from build123d import *

# Parameters (mm, degrees)
F1_DEPTH = 10
F3_DEPTH = 45
F4_W     = 2.981
F4_H     = 5
F4_W_2   = 1.6583123952
F5_DEPTH = 25
F6_R     = 2.49999
F8_DEPTH = 10
F9_R     = 2.5


# Not quite as in the source:
# - a fillet or chamfer is up to 0.001 mm smaller than in the source, because OpenCascade refuses the exact size
# - ends of sketch curves that miss each other by under 0.0002 mm in the source are joined


with BuildPart() as f1:
    # F0 (on Top) → F1 (new body)
    with BuildSketch(Plane.XY):
        with BuildLine():
            Line((70, 0), (10, 0))
            ThreePointArc((10, 0), (2.9289321881, -2.9289321881), (0, -10))
            Line((0, -10), (0, -40))
            ThreePointArc((0, -40), (2.9289321881, -47.0710678119), (10, -50))
            Line((10, -50), (70, -50))
            ThreePointArc((70, -50), (77.0710678119, -47.0710678119), (80, -40))
            Line((80, -40), (80, -10))
            ThreePointArc((80, -10), (77.0710678119, -2.9289321881), (70, 0))
        make_face()
    extrude(amount=F1_DEPTH)

    # F2 (on face) → F3 (cut)
    with BuildSketch(Plane.XZ.offset(50)):
        with BuildLine():
            ThreePointArc((40.8291561976, 0), (41.3216910184, 0.5406814173), (41.5, 1.25))
            ThreePointArc((41.5, 1.25), (39.2906814173, 2.5716910184), (39.1708438024, 0))
            Line((39.1708438024, 0), (40.8291561976, 0))
        make_face()
    extrude(amount=-F3_DEPTH, mode=Mode.SUBTRACT)

    # F4 (on face) → F5 (cut)
    with BuildSketch(Plane(origin=(0, 0, 0), x_dir=(1, 0, 0), z_dir=(0, 0, -1))):
        with Locations((37.6803438024, 7.5)):
            Rectangle(F4_W, F4_H)
        with Locations((40, 7.5)):
            Rectangle(F4_W_2, F4_H)
        with Locations((42.3196561976, 7.5)):
            Rectangle(F4_W, F4_H)
    extrude(amount=-F5_DEPTH, mode=Mode.SUBTRACT)

    # F6 (radius 2.5 in the source; OpenCascade refuses exactly that, so slightly less here)
    f6_edges = [f1.edges().sort_by_distance(p)[0] for p in [
        (36.189844, -5, 5),
        (43.810156, -5, 5),
        (43.810156, -10, 5),
        (36.189844, -10, 5),
    ]]
    fillet(f6_edges, radius=F6_R)

    # F7 (on face) → F8 (join)
    with BuildSketch(Plane.XY.offset(10)):
        Polygon((35.1898438024, -11), (40, -11), (44.8101561976, -11), (44.8101561976, -4), (35.1898438024, -4), align=None)
        with BuildLine():
            ThreePointArc((38.6898338024, -10), (36.9220739205, -9.2677698819), (36.1898438024, -7.50001))
            ThreePointArc((36.1898438024, -7.50001), (36.9220739205, -5.7322301181), (38.6898338024, -5))
            Line((38.6898338024, -5), (41.3101661976, -5))
            ThreePointArc((41.3101661976, -5), (43.0779260795, -5.7322301181), (43.8101561976, -7.49999))
            ThreePointArc((43.8101561976, -7.49999), (43.0779260795, -9.2677698819), (41.3101661976, -10))
            Line((41.3101661976, -10), (38.6898338024, -10))
        make_face(mode=Mode.SUBTRACT)
    extrude(amount=F8_DEPTH)

    # F9
    f9_edges = [f1.edges().sort_by_distance(p)[0] for p in [
        (44.810156, -4, 15),
        (35.189844, -4, 15),
        (35.189844, -11, 15),
        (44.810156, -11, 15),
    ]]
    fillet(f9_edges, radius=F9_R)


solid = f1.part
Geometry: final body of the model. Coordinates: model frame, mm. A direction names the side the tool comes from. Round coordinates to 2 decimals unless told otherwise and drop trailing zeros. Loops run counter-clockwise (first coordinate to the right, second up) from the corner with the lowest first, then second, coordinate; pieces in that order, holes last.
Q1. Pin query (flat end, axial travel): P1, Ø8, axis at y = -17.5, z = 12.5, coming from the +X side; P2, Ø3, axis at x = 39.5, z = 12.5, coming from the +Y side; P3, Ø12, axis at x = 28.5, y = -36, coming from the +Z side; P4, Ø1.6, axis at y = -7.5, z = 14, coming from the +X side. Return the tip coordinate at first contact, or that it passes through.
Q2. Section C-C on x = 9. Return loops of the section in (y, z), plus the area to 3 significant figures.
Q3. Access query for faces 4 (the cylindrical face through (35.903, -4.752, 15.07)), 5 (the cylindrical face through (35.942, -10.287, 15.07)), 6 (the flat face through (35.19, -7, 15)), 7 (the flat face through (44.81, -8, 15)), 8 (the flat face through (40, -10, 11)). Directions: +Z, -Z, +X, -X, +Y, -Y. A direction counts if a zero-diameter tool reaches every point of the face in a straight line with its end or side. Return the directions, or none.
Q4. Material intervals for L1, parallel to X at y = -29.5, z = 1.25; L2, parallel to Y at x = 40, z = 12; L3, parallel to Z at x = 40, y = -23, sorted ascending.
Q5. Section D-D on x = 72. Return loops of the section in (y, z), plus the area to 3 significant figures.
Q6. Pull-direction query (X, two-part tool) for faces 1 (the cylindrical face through (76.99, -47.15, 4.93)), 2 (the flat face through (0, -25, 5)), 3 (the cylindrical face through (36.903, -9.248, 0.263)); classes: released by +X, released by -X, zero draft, split by the parting line, or undercut.
Q7. Section A-A on x = 40. Return loops of the section in (y, z), plus the area to 3 significant figures.
Evaluation:
1. P1: stops at x = 80
1. P2: stops at y = -4
1. P3: stops at z = 10
1. P4: stops at x = 44.81
2. outline: (-49.95, 0) - (-0.05, 0) - (-0.05, 10) - (-49.95, 10) - close
2. area: 499 mm2
3. face 4: +Z, -X, +Y
3. face 5: +Z, -X, -Y
3. face 6: +Z, -X, +Y, -Y
3. face 7: +Z, +X, +Y, -Y
3. face 8: +Z, -Z
4. L1: x = 0 to 38.5, 41.5 to 80
4. L2: y = -11 to -10, -5 to -4
4. L3: z = 2.75 to 10
5. outline: (-49.8, 0) - (-0.2, 0) - (-0.2, 10) - (-49.8, 10) - close
5. area: 496 mm2
6. face 1: released by +X
6. face 2: released by -X
6. face 3: undercut
7. outline: (-50, 2.75) - (-10, 2.75) - (-10, 20) - (-11, 20) - (-11, 10) - (-50, 10) - close; (-5, 0) - (0, 0) - (0, 10) - (-4, 10) - (-4, 20) - (-5, 20) - close
7. area: 360 mm2
